from build123d import *

# Parameters (mm, degrees)
BOSS_EXTRUDE1_DEPTH = 20
SKETCH2_R           = 2.5
CUT_EXTRUDE1_DEPTH  = 15


with BuildPart() as part:
    # Sketch1 → Boss-Extrude1 (new body)
    with BuildSketch(Plane.XY):
        with BuildLine():
            Line((-5, 12.247448714), (-5, 25))
            Line((-5, 25), (0, 25))
            Line((0, 25), (0, 7.5))
            Line((0, 7.5), (-7.5, 7.5))
            ThreePointArc((-7.5, 7.5), (-15, 0), (-7.5, -7.5))
            Line((-7.5, -7.5), (0, -7.5))
            Line((0, -7.5), (0, -25))
            Line((0, -25), (-5, -25))
            Line((-5, -25), (-5, -12.247448714))
            ThreePointArc((-5, -12.247448714), (-20, 0), (-5, 12.247448714))
        make_face()
    extrude(amount=BOSS_EXTRUDE1_DEPTH)

    # Sketch2 → Cut-Extrude1 (cut)
    with BuildSketch(Plane.ZY.offset(5)):
        with Locations(Location((10, 20, 0), (0, 0, 270))):
            Circle(SKETCH2_R)
        with Locations(Location((10, -20, 0), (0, 0, 270))):
            Circle(SKETCH2_R)
    extrude(amount=-CUT_EXTRUDE1_DEPTH, mode=Mode.SUBTRACT)


solid = part.part
Could you check a few things on this model? Use its own coordinates, in mm. A direction names the side the tool comes from. Give positions to 0.01 mm unless a question says otherwise; leave off trailing zeros. Loops run counter-clockwise (first coordinate to the right, second up) from the corner with the lowest first, then second, coordinate; pieces in that order, holes last. Notation, with made-up numbers: (19, -38) -> (29, -38) arc R37 ccw to (29, -1) -> close; hole circle Ø8 at (-6, -0.75). An arc over 180 degrees is marked (long way). Return JSON: item names as keys, results as strings.
Item 1: If we section it at B-B on z = 12: List the corners of the cut face in (x, y) for me.
Geometry results:
{"outline": "(-7.5, -7.5) arc R7.5 cw to (-7.5, 7.5) -> (0, 7.5) -> (0, 18.5) -> (-5, 18.5) -> (-5, 12.25) arc R12.5 ccw (long way) to (-5, -12.25) -> (-5, -18.5) -> (0, -18.5) -> (0, -7.5) -> close; (-5, -25) -> (0, -25) -> (0, -21.5) -> (-5, -21.5) -> close; (-5, 21.5) -> (0, 21.5) -> (0, 25) -> (-5, 25) -> close"}
Item 2: Which directions (+Z, -Z, +X, -X, +Y, -Y) give clear straight access to the entire face, cutting with the end or side of a thin tool? Please do faces 5 (the flat face through (-4, -7.5, 10)), 6 (the flat face through (-3, 25, 10)).
Geometry results:
{"face 5": "+Z, -Z, +X", "face 6": "+Z, -Z, +X, -X, +Y"}
Item 3: I'm going to push flat-ended pins straight in: pin 1 (6 mm diameter, centred on x = -7, z = 18, fed in from -Y); pin 2 (4 mm diameter, centred on x = -8.5, z = 7.5, fed in from -Y); pin 3 (3 mm diameter, centred on x = -15.5, z = 2.5, fed in from +Y); pin 4 (8 mm diameter, centred on y = 20, z = 10, fed in from -X). Where does each tip first touch, or does it pass through?
Geometry results:
{"pin 1": "stops at y = -25", "pin 2": "stops at y = -12.5", "pin 3": "stops at y = 10.68", "pin 4": "stops at x = -5"}
Item 4: If we section it at A-A on y = -18.5: List the corners of the cut face in (x, z) for me, plus the area to 3 significant figures.
Geometry results:
{"outline": "(-5, 0) -> (0, 0) -> (0, 8) -> (-5, 8) -> close; (-5, 12) -> (0, 12) -> (0, 20) -> (-5, 20) -> close", "area": "80.0 mm²"}
Item 5: We'd pull the mould along Z, two halves only. Please class faces 1 (the flat face through (-2, -25, 10)), 2 (the flat face through (-8, 8, 20)), 3 (the flat face through (-8, 8, 0)), 4 (the cylindrical face through (-2.5, 22, 8.5)): +Z half, -Z half, draft (parallel to the pull), parting line (faces both ways), or undercut.
Geometry results:
{"face 1": "draft", "face 2": "+Z half", "face 3": "-Z half", "face 4": "undercut"}
Item 6: I need wall thicknesses on L1, parallel to Y at x = -3.75, z = 1; L2, parallel to Z at x = -1.4, y = 20; L3, parallel to X at y = -21, z = 1. Which ranges of each line are inside material? Lowest first, please. Write a range as from..to.
Geometry results:
{"L1": "y = -25..-7.5, 7.5..25", "L2": "z = 0..7.5, 12.5..20", "L3": "x = -5..0"}
Item 7: If we section it at D-D on z = 15.5: List the corners of the cut face in (x, y) for me, plus the area to 3 significant figures.
Geometry results:
{"outline": "(-7.5, -7.5) arc R7.5 cw to (-7.5, 7.5) -> (0, 7.5) -> (0, 25) -> (-5, 25) -> (-5, 12.25) arc R12.5 ccw (long way) to (-5, -12.25) -> (-5, -25) -> (0, -25) -> (0, -7.5) -> close", "area": "357 mm²"}
Item 8: If we section it at C-C on x = -10.75: List the corners of the cut face in (y, z) for me.
Geometry results:
{"outline": "(-12.07, 0) -> (-6.76, 0) -> (-6.76, 20) -> (-12.07, 20) -> close; (6.76, 0) -> (12.07, 0) -> (12.07, 20) -> (6.76, 20) -> close"}
